Geometry: final body of the model. Coordinates: model frame, mm. A direction names the side the tool comes from. Coordinates: 2 decimals unless noted, no trailing zeros. Write each loop counter-clockwise with the first axis right and the second up, starting at its lowest first coordinate (ties: lowest second). Pieces come first, ordered by that corner, then holes.
from build123d import *

# Parameters (mm, degrees)
SKETCH1_R           = 12.4
BOSS_EXTRUDE1_DEPTH = 5
SKETCH2_R           = 7.3
BOSS_EXTRUDE2_DEPTH = 69
SKETCH3_R           = 2.7
CUT_EXTRUDE1_DEPTH  = 75
CUT_EXTRUDE2_DEPTH  = 3
FILLET1_R           = 0.5


with BuildPart() as part:
    # Sketch1 → Boss-Extrude1 (new body)
    with BuildSketch(Plane(origin=(0, 0, 0), x_dir=(1, 0, 0), z_dir=(0, 1, 0))):
        Circle(SKETCH1_R)
    extrude(amount=BOSS_EXTRUDE1_DEPTH)

    # Sketch2 → Boss-Extrude2 (add)
    with BuildSketch(Plane(origin=(0, 5, 0), x_dir=(1, 0, 0), z_dir=(0, 1, 0))):
        Circle(SKETCH2_R)
    extrude(amount=BOSS_EXTRUDE2_DEPTH)

    # Sketch3 → Cut-Extrude1 (cut, through all)
    with BuildSketch(Plane(origin=(0, 74, 0), x_dir=(1, 0, 0), z_dir=(0, 1, 0))):
        Circle(SKETCH3_R)
    extrude(amount=-CUT_EXTRUDE1_DEPTH, mode=Mode.SUBTRACT)

    # Sketch4 → Cut-Extrude2 (cut)
    with BuildSketch(Plane.XZ):
        Polygon((-4.38019792, 2.081793981), (-3.992985433, -2.752465682), (0.387212487, -4.834259663), (4.38019792, -2.081793981), (3.992985433, 2.752465682), (-0.387212487, 4.834259663), align=None)
    extrude(amount=-CUT_EXTRUDE2_DEPTH, mode=Mode.SUBTRACT)

    # Fillet1
    fillet1_edges = [part.edges().sort_by_distance(p)[0] for p in [
        (-12.4, 0, 0),
        (-12.4, 5, 0),
        (-7.3, 5, 0),
        (-7.3, 74, 0),
    ]]
    fillet(fillet1_edges, radius=FILLET1_R)


solid = part.part
Item 1: Section A-A, the plane z = 0. Output: boundary loops of the cut face in (x, y), plus the area to 3 significant figures.
Derived:
outline: (-12.4, 0.5) arc R0.5 ccw to (-11.9, 0) - (-4.21, 0) - (-4.21, 3) - (-2.7, 3) - (-2.7, 74) - (-6.8, 74) arc R0.5 ccw to (-7.3, 73.5) - (-7.3, 5.5) arc R0.5 cw to (-7.8, 5) - (-11.9, 5) arc R0.5 ccw to (-12.4, 4.5) - close; (2.7, 3) - (4.21, 3) - (4.21, 0) - (11.9, 0) arc R0.5 ccw to (12.4, 0.5) - (12.4, 4.5) arc R0.5 ccw to (11.9, 5) - (7.8, 5) arc R0.5 cw to (7.3, 5.5) - (7.3, 73.5) arc R0.5 ccw to (6.8, 74) - (2.7, 74) - close
area: 723 mm2
Item 2: Set-up query: faces 4 (the flat face through (2.356, 1.479, -3.477)), 5 (the flat face through (5, 0, 0)). Return all of +Z, -Z, +X, -X, +Y, -Y with unobstructed straight access to the full face (end or side cutting, diameter ignored); none if empty.
Derived:
face 4: -Y
face 5: +Z, -Z, +X, -X, -Y
Item 3: Material intervals for probe 1 along Z at (x, y) = (0, 28); probe 2 along Y at (x, z) = (5, -8), sorted ascending.
Derived:
probe 1: z = -7.3 to -2.7, 2.7 to 7.3
probe 2: y = 0 to 5
Item 4: Pull-direction query (Z, two-part tool) for faces 1 (the flat face through (8, 5, 2)), 2 (the cylindrical face through (6.963, 39.024, -2.193)), 3 (the flat face through (1.83, 1.48, 3.78)); classes: released by +Z, released by -Z, zero draft, split by the parting line, or undercut.
Derived:
face 1: zero draft
face 2: split by the parting line
face 3: undercut
Item 5: Pin query (flat end, axial travel): pin 1 (4 mm diameter, centred on x = -1, z = 8.5, fed in from +Y); pin 2 (6 mm diameter, centred on x = 5.5, y = 49.5, fed in from -Z); pin 3 (8 mm diameter, centred on x = -0.5, y = 32.5, fed in from -Z); pin 4 (8 mm diameter, centred on y = 55.5, z = 6.5, fed in from -X). Return the tip coordinate at first contact, or that it passes through.
Derived:
pin 1: stops at y = 74
pin 2: stops at z = -6.86
pin 3: stops at z = -7.3
pin 4: stops at x = -6.86
Item 6: Section B-B, the plane y = 17.5. Output: boundary loops of the cut face in (x, z).
Derived:
outline: circle Ø14.6 at (0, 0); hole circle Ø5.4 at (0, 0)
